```python
from build123d import *

# Parameters (mm, degrees)
F1_DEPTH = 11.1125
F2_R     = 2.54
F3_R     = 2.4765
F4_DEPTH = 5.08
F5_W     = 25.4
F5_H     = 22.225
F5_R     = 7.9375
F6_DEPTH = 3.81


# Not quite as in the source:
# - a fillet or chamfer that OpenCascade refuses, or shapes differently, is made with other operations: its cross-section is extruded or revolved along the edge and cut away or added


with BuildPart() as f1:
    # F0 (on Front) → F1 (new body, symmetric)
    with BuildSketch(Plane.XZ):
        Polygon((-4.490128064, 4.490128064), (-12.7, 12.7), (-12.7, -12.7), (12.7, -12.7), (12.7, 12.7), (4.4901280734, 4.4901280734), (0, 0), align=None)
        with BuildLine():
            ThreePointArc((4.4901280734, 4.4901280734), (6.6e-09, 2.6302561211), (-4.490128064, 4.490128064))
            Line((-4.490128064, 4.490128064), (0, 0))
            Line((0, 0), (4.4901280734, 4.4901280734))
        make_face()
    extrude(amount=F1_DEPTH, both=True)

    # F2
    f2_edges = [f1.edges().sort_by_distance(p)[0] for p in [
        (12.7, 0, 12.7),
        (-12.7, 0, 12.7),
    ]]
    fillet(f2_edges, radius=F2_R)

    # F3 (on face) → F4 (cut)
    with BuildSketch(Plane(origin=(0, 0, -12.7), x_dir=(1, 0, 0), z_dir=(0, 0, -1))):
        Circle(F3_R)
    extrude(amount=-F4_DEPTH, mode=Mode.SUBTRACT)

    # F5 (on face) → F6 (cut)
    with BuildSketch(Plane(origin=(0, 0, -12.7), x_dir=(1, 0, 0), z_dir=(0, 0, -1))):
        Rectangle(F5_W, F5_H)
        Circle(F5_R, mode=Mode.SUBTRACT)
    extrude(amount=-F6_DEPTH, mode=Mode.SUBTRACT)

    # F7: chamfer of 5.08 on 1 edges, made by hand


with BuildPart() as f7_tool2:
    # F7_s3 → F7_t4 (revolve)
    with BuildSketch(Plane.XZ):
        Polygon((13.0175, -8.89), (7.9375, -13.97), (7.9375, -8.89), align=None)
    revolve(axis=Axis((0, 0, -8.89), (0, 0, -1)))

    split(bisect_by=Plane.XZ.offset(-11.1125), keep=Keep.TOP)

    split(bisect_by=Plane.XZ.offset(11.1125), keep=Keep.BOTTOM)

    split(bisect_by=Plane.YZ.offset(12.7), keep=Keep.BOTTOM)

    split(bisect_by=Plane.YZ.offset(-12.7), keep=Keep.TOP)

    split(bisect_by=Plane.XY.offset(-12.7), keep=Keep.TOP)


with BuildPart() as f1_1:
    add(f1.part)

    # F7_t1: union F7_tool2
    add(f7_tool2.part)


solid = f1_1.part
```
Build history of the part. All positions in model axes, mm. A direction names the side the tool comes from. Round coordinates to 2 decimals unless told otherwise and drop trailing zeros. Loops run counter-clockwise (first coordinate to the right, second up) from the corner with the lowest first, then second, coordinate; pieces in that order, holes last.
Item 1: Saw through at B-B (x = 0). List the corners of the cut face in (y, z) (1 decimal).
Item 2: Drill centre lines: line 1 along Y through (x, z) = (0, -8.7); line 2 along X through (y, z) = (0, -8.7); line 3 along X through (y, z) = (-7.25, 6.75). Where is each one in solid material? Low to high.
Item 3: Two-plate mould, pull along Y, no slides. Class faces 6 (the face through (8.959, -2.821, -12.515)), 7 (the face through (11, -9, -8.89)), 8 (the face through (0, -11.112, -1)), 9 (the face through (-0.322, -2.455, -10.196)): released by +Y, released by -Y, zero draft, split by the parting line, or undercut.
Item 4: Which spindle directions (+Z, -Z, +X, -X, +Y, -Y) get a long thin tool onto all of the face, cutting with end or side? Do faces 1 (the face through (11, 9, -8.89)), 2 (the face through (-11, -9, -8.89)), 3 (the face through (-11, 9, -8.89)), 4 (the face through (0, 0, -7.62)), 5 (the face through (-6, 0, 6)). Say none if no direction does.
Item 5: Saw through at D-D (y = 0). List the corners of the cut face in (x, z), then the cut area to 3 significant figures.
Item 6: Saw through at A-A (z = 5.5). List the corners of the cut face in (x, y).
Item 7: Saw through at C-C (z = -8.5). List the corners of the cut face in (x, y).
Item 8: Pin check, flat tips, straight feed: P1, Ø8, axis at x = -5, y = 8.5, coming from the +Z side; P2, Ø4.5, axis at x = -9, y = -9, coming from the -Z side; P3, Ø8, axis at x = 0, y = 0, coming from the +Z side. Stop position of each tip, or through.
Worked answers:
1. outline: (-11.1, -10.8) - (-9.2, -12.7) - (-2.5, -12.7) - (-2.5, -7.6) - (2.5, -7.6) - (2.5, -12.7) - (9.2, -12.7) - (11.1, -10.8) - (11.1, 2.6) - (-11.1, 2.6) - close
2. line 1: y = -11.11 to -2.48, 2.48 to 11.11
2. line 2: x = -12.7 to -2.48, 2.48 to 12.7
2. line 3: x = -12.69 to -6.75, 6.75 to 12.69
3. face 6: split by the parting line
3. face 7: zero draft
3. face 8: released by -Y
3. face 9: undercut
4. face 1: -Z, +X, +Y
4. face 2: -Z, -X, -Y
4. face 3: -Z, -X, +Y
4. face 4: -Z
4. face 5: +Z, +Y, -Y
5. outline: (-12.7, -9.21) - (-9.21, -12.7) - (-2.48, -12.7) - (-2.48, -7.62) - (2.48, -7.62) - (2.48, -12.7) - (9.21, -12.7) - (12.7, -9.21) - (12.7, 6.57) arc R2.54 ccw to (8.36, 8.36) - (4.49, 4.49) arc R6.35 cw to (-4.49, 4.49) - (-8.36, 8.36) arc R2.54 ccw to (-12.7, 6.57) - close
5. area: 439 mm2
6. outline: (-12.7, -11.11) - (-5.5, -11.11) - (-5.5, 11.11) - (-12.7, 11.11) - close; (5.5, -11.11) - (12.7, -11.11) - (12.7, 11.11) - (5.5, 11.11) - close
7. outline: (-12.7, -11.11) - (12.7, -11.11) - (12.7, 11.11) - (-12.7, 11.11) - close; hole circle Ø4.95 at (0, 0)
8. P1: stops at z = 8.83
8. P2: stops at z = -11.43
8. P3: stops at z = 4.05
